Design review of the part built by this model. Coordinates are the model's own, in mm. A direction names the side the tool comes from. Give positions to 0.01 mm unless a question says otherwise; leave off trailing zeros. Loops run counter-clockwise (first coordinate to the right, second up) from the corner with the lowest first, then second, coordinate; pieces in that order, holes last. Notation, with made-up numbers: M 26.25,-32 L 38.25,-32 A18 ccw 38.25,-2 Z; hole C -14,56 d9. An arc over 180 degrees is marked long. Use a Markdown table: item, result. Add a question column.
(1) Draft analysis for pull direction Z (two halves, no side actions). For faces 6 (the face through (25.044, -30.164, 28.6)), 7 (the face through (154.53, -20.44, 43.27)), 8 (the face through (225.15, -3.13, 4.2)), 9 (the face through (304.8, -20, 8)), state which applies: pulls with the +Z half, pulls with the -Z half, needs draft (parallel to the pull), parting line crosses it, or undercut.
(2) Add section D-D, the plane x = 142. Give the boundary of the cut face in (y, z) (3 decimals).
(3) For probe 1 along Y at (x, z) = (285, 4.5) (3 decimals); probe 2 along Y at (x, z) = (24, 40) (3 decimals); probe 3 along Z at (x, y) = (63, -23), list the stretches that pass through material, from the lowest coordinate up.
(4) Insertion check: pin 1 Ø6 at (y, z) = (-20.5, 28) entering from -X; pin 2 Ø10 at (x, y) = (222.5, -25) entering from +Z; pin 3 Ø3 at (x, y) = (164, -17) entering from +Z. Each pin has a flat end and moves straight along its axis. Give the tip position at first contact, or say it passes through.
(5) Add section B-B, the plane y = -26. Give the boundary of the cut face in (x, z) (1 decimal), then the cut area to 3 significant figures.
(6) For faces 1 (the face through (0, -20, 44)), 2 (the face through (50.8, -20, 33)), 3 (the face through (112.775, -38.144, 45.007)), 4 (the face through (225.15, -38.14, 4.2)), 5 (the face through (112.775, -3.131, 45.007)), list the 3-axis set-ups (+Z, -Z, +X, -X, +Y, -Y) from which the entire face can be reached by the end or side of a thin tool; tool diameter is ignored.
(7) Add section C-C, the plane z = 29.5. Give the boundary of the cut face in (x, y) (3 decimals), then the cut area to 3 significant figures.
```python
from build123d import *

# Parameters (mm, degrees)
F1_DEPTH = 41.275
F2_R     = 10.3124
F3_DEPTH = 50.8
F5_DEPTH = 6.35


# Not quite as in the source:
# - a pattern or mirror of a feature is missing from the dataset's text; its kind, count and spacing are read off the source's solid


with BuildPart() as f1:
    # F0 (on Front) → F1 (new body)
    with BuildSketch(Plane.XZ):
        Polygon((0, 71.4375), (0, 0), (304.8, 0), (304.8, 15.875), align=None)
    extrude(amount=F1_DEPTH)

    # F2 (on face) → F3 (cut)
    with BuildSketch(Plane(origin=(0, 0, 0), x_dir=(0, -1, 0), z_dir=(-1, 0, 0))):
        with Locations((20.6375, 32.5501)):
            Circle(F2_R)
    extrude(amount=-F3_DEPTH, mode=Mode.SUBTRACT)

    # F4 (on face) → F5 (cut)
    with BuildSketch(Plane.XZ.offset(41.275)):
        with BuildLine():
            Line((0, 71.4375), (0, 35.71875))
            ThreePointArc((0, 35.71875), (114.380623494, 44.8132958518), (223.1006332012, 8.1309120088))
            ThreePointArc((223.1006332012, 8.1309120088), (225.1513542681, 4.1369059415), (223.4067767859, 0))
            Line((223.4067767859, 0), (304.8, 0))
            Line((304.8, 0), (304.8, 7.9375))
            Line((304.8, 7.9375), (304.8, 15.875))
            Line((304.8, 15.875), (0, 71.4375))
        make_face()
    f5 = extrude(amount=-F5_DEPTH, mode=Mode.SUBTRACT)

    # F5_copies: F5 across plane
    add(f5.mirror(Plane.ZX.offset(-20.6375)), mode=Mode.SUBTRACT)


solid = f1.part
```
Established:
| question | item | result |
|---|---|---|
| 1 | face 6 | undercut |
| 1 | face 7 | pulls with the +Z half |
| 1 | face 8 | parting line crosses it |
| 1 | face 9 | needs draft |
| 2 | outline | M -41.275,0 L 0,0 L 0,40.011 L -6.35,40.011 L -6.35,45.552 L -34.925,45.552 L -34.925,40.011 L -41.275,40.011 Z |
| 3 | probe 1 | -34.925 to -6.35 |
| 3 | probe 2 | -41.275 to -27.768, -13.507 to 0 |
| 3 | probe 3 | 0 to 59.95 |
| 4 | pin 1 | x = 50.8 |
| 4 | pin 2 | z = 31.79 |
| 4 | pin 3 | z = 41.82 |
| 5 | outline | M 0,0 L 304.8,0 L 304.8,15.9 L 0,71.4 L 0,41.4 L 50.8,41.4 L 50.8,23.7 L 0,23.7 Z |
| 5 | area | 12,400 mm^2 |
| 6 | face 1 | +Z, -Z, -X, +Y, -Y |
| 6 | face 2 | -X |
| 6 | face 3 | +Z, -Y |
| 6 | face 4 | +X, -Y |
| 6 | face 5 | +Z, +Y |
| 7 | outline | M 0,-41.275 L 177.679,-41.275 L 177.679,-34.925 L 230.057,-34.925 L 230.057,-6.35 L 177.679,-6.35 L 177.679,0 L 0,0 L 0,-10.786 L 50.8,-10.786 L 50.8,-30.489 L 0,-30.489 Z |
| 7 | area | 7,830 mm^2 |
